Could you check a few things on this model? Use its own coordinates, in mm. A direction names the side the tool comes from. Coordinates: 2 decimals unless noted, no trailing zeros. Order: outer loops, then holes, each group sorted by start corner. A loop starts at its lowest first (then second) coordinate and runs counter-clockwise, first axis right, second up. Notation, with made-up numbers: (87, 52.25) -> (107, 52.25) arc R10 cw to (107, 62.25) -> close; hole circle Ø2 at (71, 66). An arc over 180 degrees is marked (long way). Use a Markdown table: item, result. Add a question column.
1) Will these pins go through, and if not, where does the flat tip stop? pin 1 Ø5 at (y, z) = (-13, 10.5) entering from -X; pin 2 Ø10 at (y, z) = (-48, -24) entering from -X; pin 3 Ø12 at (y, z) = (-48, -9.5) entering from +X.
2) Thinking about a two-plate mould opening in X: for faces 4 (the flat face through (30, -34.8, 0.3)), 5 (the cylindrical face through (-35.015, -0.21, 0.66)), 6 (the flat face through (1, 0, 30)), which applies, +X half, -X half, draft (parallel to the pull), parting line (faces both ways), or undercut?
3) Which directions (+Z, -Z, +X, -X, +Y, -Y) give clear straight access to the entire face, cutting with the end or side of a thin tool? Please do faces 1 (the flat face through (15.288, -56, 0)), 2 (the flat face through (-30, -34, 0)), 3 (the flat face through (0, -26, -20)).
4) If we section it at A-A (x = -42): Write out the boundary of the cut face in (y, z), plus the area to 3 significant figures.
5) If we section it at C-C (y = -19): Write out the boundary of the cut face in (x, z).
6) If I drill on L1, parallel to Z at x = -50, y = 1.5; L2, parallel to X at y = 10, z = -12; L3, parallel to Y at x = 49.5, z = -17, over which ranges is the centre line in solid material (lowest first)? Write a range as [from, to].
7) If we section it at B-B (x = 0): Write out the boundary of the cut face in (y, z), plus the area to 3 significant figures.
```python
from build123d import *

# Parameters (mm, degrees)
F1_DEPTH = 15
F3_DEPTH = 20
F5_DEPTH = 110.001
F7_DEPTH = 110.001


with BuildPart() as f1:
    # F0 (on Front) → F1 (new body, symmetric)
    with BuildSketch(Plane.XZ):
        with BuildLine():
            Line((35, 0), (-35, 0))
            ThreePointArc((-35, 0), (-50, -15), (-65, 0))
            Line((-65, 0), (-80, 0))
            ThreePointArc((-80, 0), (-71.2132034356, -21.2132034356), (-50, -30))
            Line((-50, -30), (50, -30))
            ThreePointArc((50, -30), (71.2132034356, -21.2132034356), (80, 0))
            Line((80, 0), (65, 0))
            ThreePointArc((65, 0), (50, -15), (35, 0))
        make_face()
        with BuildLine():
            ThreePointArc((-65, 0), (-50, 15), (-35, 0))
            Line((-35, 0), (35, 0))
            ThreePointArc((35, 0), (50, 15), (65, 0))
            Line((65, 0), (80, 0))
            ThreePointArc((80, 0), (71.2132034356, 21.2132034356), (50, 30))
            Line((50, 30), (-50, 30))
            ThreePointArc((-50, 30), (-71.2132034356, 21.2132034356), (-80, 0))
            Line((-80, 0), (-65, 0))
        make_face()
    extrude(amount=F1_DEPTH, both=True)

    # F2 (on Top) → F3 (join, symmetric)
    with BuildSketch(Plane.XY):
        with BuildLine():
            Line((-30, -15), (-30, -65))
            Line((-30, -65), (-15.0350227241, -65))
            Line((-15.0350227241, -65), (-15.0350227241, -44.9706647246))
            ThreePointArc((-15.0350227241, -44.9706647246), (-15.3514603972, -41.869789362), (-15.0350227241, -38.7689139994))
            ThreePointArc((-15.0350227241, -38.7689139994), (0.8607482539, -26.5424788095), (15.2876708067, -40.4717701802))
            ThreePointArc((15.2876708067, -40.4717701802), (15.3514603972, -41.869789362), (15.2876708067, -43.2678085437))
            Line((15.2876708067, -43.2678085437), (15.2876708067, -65))
            Line((15.2876708067, -65), (30, -65))
            Line((30, -65), (30, -15))
            Line((30, -15), (-30, -15))
        make_face()
    extrude(amount=F3_DEPTH, both=True)

    # F4 (on face) → F5 (cut, through all)
    with BuildSketch(Plane(origin=(-30, 0, 0), x_dir=(0, -1, 0), z_dir=(-1, 0, 0))):
        with BuildLine():
            Line((65, 20), (45, 20))
            ThreePointArc((45, 20), (59.1421356638, 14.1421355837), (65, -1.132e-07))
            Line((65, -1.132e-07), (65, 20))
        make_face()
        with BuildLine():
            ThreePointArc((65, -1.132e-07), (59.1421355837, -14.1421356638), (45, -20))
            Line((45, -20), (65, -20))
            Line((65, -20), (65, -1.132e-07))
        make_face()
    extrude(amount=-F5_DEPTH, mode=Mode.SUBTRACT)

    # F6 (on face) → F7 (cut, through all)
    with BuildSketch(Plane(origin=(-30, 0, 0), x_dir=(0, -1, 0), z_dir=(-1, 0, 0))):
        with BuildLine():
            ThreePointArc((55, 0), (52.0710678119, 7.0710678119), (45, 10))
            Line((45, 10), (45, -10))
            ThreePointArc((45, -10), (52.0710678119, -7.0710678119), (55, 0))
        make_face()
        with BuildLine():
            Line((45, -10), (45, 10))
            ThreePointArc((45, 10), (35, 0), (45, -10))
        make_face()
    extrude(amount=-F7_DEPTH, mode=Mode.SUBTRACT)


solid = f1.part
```
Answer sheet:
| question | item | result |
|---|---|---|
| 1 | pin 1 | x = -78.91 |
| 1 | pin 2 | x = -30 |
| 1 | pin 3 | x = 30 |
| 2 | face 4 | +X half |
| 2 | face 5 | undercut |
| 2 | face 6 | draft |
| 3 | face 1 | +Z, -Z, -Y |
| 3 | face 2 | +Z, -Z, -X, -Y |
| 3 | face 3 | -Z, +X, -X, -Y |
| 4 | outline | (-15, -30) -> (15, -30) -> (15, -12.69) -> (-15, -12.69) -> close; (-15, 12.69) -> (15, 12.69) -> (15, 30) -> (-15, 30) -> close |
| 4 | area | 1,040 mm2 |
| 5 | outline | (-30, -20) -> (30, -20) -> (30, 20) -> (-30, 20) -> close |
| 6 | L1 | [-30, -15], [15, 30] |
| 6 | L2 | [-77.5, -59], [-41, 41], [59, 77.5] |
| 6 | L3 | [-15, 15] |
| 7 | outline | (-26.52, -20) -> (-15, -20) -> (-15, -30) -> (15, -30) -> (15, 30) -> (-15, 30) -> (-15, 20) -> (-26.52, 20) -> close |
| 7 | area | 2,260 mm2 |
